Answer from the drawing. Dimensions are ordinates in mm from the lowest x, y and z of the part. A direction names the side the tool comes from. Round coordinates to 2 decimals unless told otherwise and drop trailing zeros. Loops run counter-clockwise (first coordinate to the right, second up) from the corner with the lowest first, then second, coordinate; pieces in that order, holes last. Notation, with made-up numbers: (76.5, 24.5) - (133.5, 24.5) arc R9 cw to (133.5, 32.5) - close; hole circle Ø10 at (55.5, -33). An arc over 180 degrees is marked (long way). Write item = value, one per line. Start each with the question number.
1) Section D-D, the plane y = 15.5 is taken. Determine the outline of the cut face in (x, z), and give its area (3 significant figures).
2) Given pin 1 Ø4.5 at (x, z) = (92, 105.5) entering from -Y; pin 2 Ø3 at (x, z) = (55, 80.5) entering from +Y, each flat-ended and moving along its own axis, determine where each tip first touches the part or whether it passes through.
3) Section B-B, the plane x = 81 is taken. Determine the outline of the cut face in (y, z).
4) Straight lines are drawn through the part: line 1 along X through (y, z) = (14.5, 32); line 2 along Z through (x, y) = (19, 34); line 3 along Y through (x, z) = (54, 53). For each, find the intervals that lie inside material, in ascending order.
5) Section A-A, the plane z = 59.5 is taken. Determine the outline of the cut face in (x, y).
6) For a pull along X with two mould halves and no side action, classify the marked faces 1, 2, 3 and 4 as released by +X, released by -X, zero draft, split by the parting line, or undercut.
7) Section C-C, the plane y = 66 is taken. Determine the outline of the cut face in (x, z).
8) A tool of negligible diameter and unlimited length cuts with its end or side. For the marked faces 5 and 6, from which of +Z, -Z, +X, -X, +Y, -Y can it reach the whole face along a straight path? Write none if from no direction.
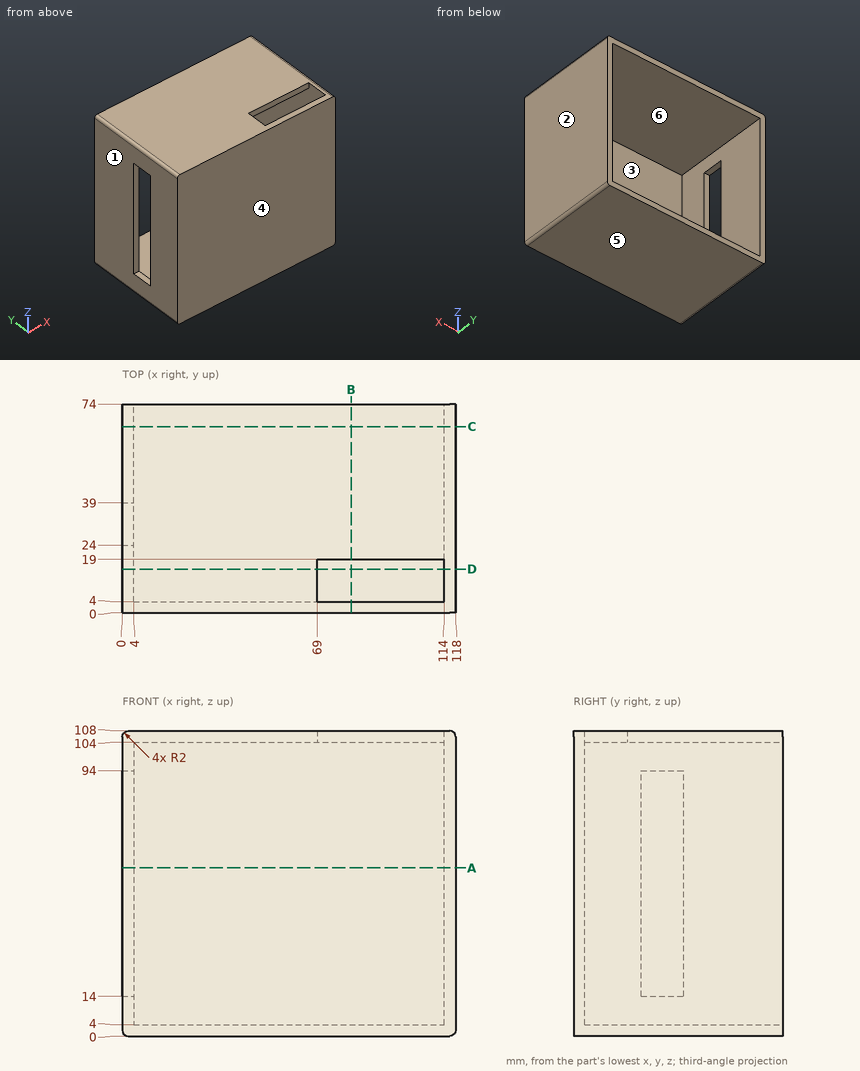
Geometry check:
q1.outline = (0, 2) arc R2 ccw to (2, 0) - (116, 0) arc R2 ccw to (118, 2) - (118, 106) arc R2 ccw to (116, 108) - (114, 108) - (114, 4) - (4, 4) - (4, 104) - (69, 104) - (69, 108) - (2, 108) arc R2 ccw to (0, 106) - close
q1.area = 1,560 mm2
q2.pin_1 = 0
q2.pin_2 = 4
q3.outline = (0, 0) - (74, 0) - (74, 4) - (4, 4) - (4, 108) - (0, 108) - close; (19, 104) - (74, 104) - (74, 108) - (19, 108) - close
q4.line_1 = 0 to 4, 114 to 118
q4.line_2 = 0 to 4, 104 to 108
q4.line_3 = 0 to 4
q5.outline = (0, 0) - (118, 0) - (118, 74) - (114, 74) - (114, 4) - (4, 4) - (4, 24) - (0, 24) - close; (0, 39) - (4, 39) - (4, 74) - (0, 74) - close
q6.face_1 = released by -X
q6.face_2 = released by +X
q6.face_3 = undercut
q6.face_4 = zero draft
q7.outline = (0, 2) arc R2 ccw to (2, 0) - (116, 0) arc R2 ccw to (118, 2) - (118, 106) arc R2 ccw to (116, 108) - (2, 108) arc R2 ccw to (0, 106) - close; hole (4, 4) - (114, 4) - (114, 104) - (4, 104) - close
q8.face_5 = -Z, +X, -X, +Y, -Y
q8.face_6 = +Y
